Design review of the part built by this model. Coordinates are the model's own, in mm. A direction names the side the tool comes from. Coordinates: 2 decimals unless noted, no trailing zeros. Loops run counter-clockwise (first coordinate to the right, second up) from the corner with the lowest first, then second, coordinate; pieces in that order, holes last. Notation, with made-up numbers: (58.25, -18) -> (63.25, -18) arc R28 cw to (63.25, 6) -> close; hole circle Ø8 at (84, 42). An arc over 180 degrees is marked (long way). Answer in a Markdown table with one row per item.
```python
from build123d import *

# Parameters (mm, degrees)
ESQUISSE1_W             = 220
ESQUISSE1_H             = 220
ESQUISSE1_R             = 2
BOSS_EXTRU_1_DEPTH      = 4
ESQUISSE2_W             = 50
ESQUISSE2_H             = 50
ENL_V_MAT_EXTRU_1_DEPTH = 5
CONG_1_R                = 5
CHANFREIN1_SIZE         = 3
CONG_2_R                = 5


with BuildPart() as part:
    # Esquisse1 → Boss.-Extru.1 (new body)
    with BuildSketch(Plane.XY):
        with Locations((-21.875157945, -21.770833333)):
            Rectangle(ESQUISSE1_W, ESQUISSE1_H)
        with Locations((-126.875157945, 83.229166667)):
            Circle(ESQUISSE1_R, mode=Mode.SUBTRACT)
        with Locations((83.124842055, 83.229166667)):
            Circle(ESQUISSE1_R, mode=Mode.SUBTRACT)
        with Locations((-126.875157945, -126.770833333)):
            Circle(ESQUISSE1_R, mode=Mode.SUBTRACT)
        with Locations((83.124842055, -126.770833333)):
            Circle(ESQUISSE1_R, mode=Mode.SUBTRACT)
        with Locations((-113.375157945, -16.770833333)):
            Circle(ESQUISSE1_R, mode=Mode.SUBTRACT)
        with Locations((-98.375157945, -16.770833333)):
            Circle(ESQUISSE1_R, mode=Mode.SUBTRACT)
        with Locations((-113.375157945, -26.770833333)):
            Circle(ESQUISSE1_R, mode=Mode.SUBTRACT)
        with Locations((-98.375157945, -26.770833333)):
            Circle(ESQUISSE1_R, mode=Mode.SUBTRACT)
        with Locations((54.624842055, -16.770833333)):
            Circle(ESQUISSE1_R, mode=Mode.SUBTRACT)
        with Locations((69.624842055, -16.770833333)):
            Circle(ESQUISSE1_R, mode=Mode.SUBTRACT)
        with Locations((54.624842055, -26.770833333)):
            Circle(ESQUISSE1_R, mode=Mode.SUBTRACT)
        with Locations((69.624842055, -26.770833333)):
            Circle(ESQUISSE1_R, mode=Mode.SUBTRACT)
        with Locations((-21.875157945, -1.270833333)):
            Circle(ESQUISSE1_R, mode=Mode.SUBTRACT)
        with Locations((-21.875157945, -42.270833333)):
            Circle(ESQUISSE1_R, mode=Mode.SUBTRACT)
    extrude(amount=BOSS_EXTRU_1_DEPTH)

    # Esquisse2 → Enlèv. mat.-Extru.1 (cut, through all)
    with BuildSketch(Plane.XY.offset(4)):
        Polygon((-89.375157945, 53.229166667), (45.624842055, 53.229166667), (5.624842055, 13.229166667), (-49.375157945, 13.229166667), align=None)
        Polygon((-89.375157945, -96.770833333), (45.624842055, -96.770833333), (5.624842055, -56.770833333), (-49.375157945, -56.770833333), align=None)
        Polygon((88.124842055, -41.770833333), (58.124842055, -71.770833333), (58.124842055, -91.770833333), (88.124842055, -121.770833333), align=None)
        Polygon((88.124842055, 78.229166667), (88.124842055, -1.770833333), (58.124842055, 28.229166667), (58.124842055, 48.229166667), align=None)
        Polygon((-131.875157945, 78.229166667), (-131.875157945, -1.770833333), (-101.875157945, 28.229166667), (-101.875157945, 48.229166667), align=None)
        Polygon((-131.875157945, -41.770833333), (-101.875157945, -71.770833333), (-101.875157945, -91.770833333), (-131.875157945, -121.770833333), align=None)
        with Locations((18.124842055, -21.770833333)):
            Rectangle(ESQUISSE2_W, ESQUISSE2_H)
        with Locations((-61.875157945, -21.770833333)):
            Rectangle(ESQUISSE2_W, ESQUISSE2_H)
        Polygon((-121.875157945, -131.770833333), (-86.171457776, -106.770833333), (42.421141887, -106.770833333), (78.124842055, -131.770833333), align=None)
        Polygon((-121.875157945, 88.229166667), (-86.171457776, 63.229166667), (42.421141887, 63.229166667), (78.124842055, 88.229166667), align=None)
    extrude(amount=-ENL_V_MAT_EXTRU_1_DEPTH, mode=Mode.SUBTRACT)

    # Congé1
    cong_1_edges = [part.edges().sort_by_distance(p)[0] for p in [
        (-89.375157945, 53.229166667, 2),
        (45.624842055, 53.229166667, 2),
        (-89.375157945, -96.770833333, 2),
        (45.624842055, -96.770833333, 2),
    ]]
    fillet(cong_1_edges, radius=CONG_1_R)

    # Chanfrein1
    chanfrein1_edges = [part.edges().sort_by_distance(p)[0] for p in [
        (-131.875157945, 88.229166667, 2),
        (88.124842055, 88.229166667, 2),
        (88.124842055, -131.770833333, 2),
        (-131.875157945, -131.770833333, 2),
    ]]
    chamfer(chanfrein1_edges, length=CHANFREIN1_SIZE)

    # Congé2
    cong_2_edges = [part.edges().sort_by_distance(p)[0] for p in [
        (58.124842055, -91.770833333, 2),
        (58.124842055, -71.770833333, 2),
        (58.124842055, 48.229166667, 2),
        (58.124842055, 28.229166667, 2),
        (-101.875157945, 48.229166667, 2),
        (-101.875157945, 28.229166667, 2),
        (-101.875157945, -71.770833333, 2),
        (-101.875157945, -91.770833333, 2),
        (-86.875157945, -46.770833333, 2),
        (-86.875157945, 3.229166667, 2),
        (-36.875157945, 3.229166667, 2),
        (-36.875157945, -46.770833333, 2),
        (-6.875157945, -46.770833333, 2),
        (-6.875157945, 3.229166667, 2),
        (43.124842055, 3.229166667, 2),
        (43.124842055, -46.770833333, 2),
        (-86.171457776, -106.770833333, 2),
        (42.421141887, -106.770833333, 2),
        (42.421141887, 63.229166667, 2),
        (-86.171457776, 63.229166667, 2),
        (-49.375157945, 13.229166667, 2),
        (5.624842055, 13.229166667, 2),
        (-49.375157945, -56.770833333, 2),
        (5.624842055, -56.770833333, 2),
    ]]
    fillet(cong_2_edges, radius=CONG_2_R)


solid = part.part
```
(1) Tool access review of faces 5 (the flat face through (74.057, 12.297, 2.028)), 6 (the flat face through (-104.91, -119.89, 2.03)), 7 (the cylindrical face through (41.699, 1.726, 1.972)), 8 (the flat face through (-104.91, 76.35, 2.03)), 9 (the flat face through (-117.408, 63.762, 2.028)): name each direction out of +Z, -Z, +X, -X, +Y, -Y from which nothing blocks a thin tool from reaching the whole face with its end or side.
Evaluation:
| item | result |
|---|---|
| face 5 | +Z, -Z, +X |
| face 6 | +Z, -Z, -Y |
| face 7 | +Z, -Z |
| face 8 | +Z, -Z, +Y |
| face 9 | +Z, -Z, -X |
(2) Take a section at D-D on x = 15. Give the boundary of the cut face in (y, z).
Evaluation:
| item | result |
|---|---|
| outline | (-106.77, 0) -> (-96.77, 0) -> (-96.77, 4) -> (-106.77, 4) -> close; (-66.15, 0) -> (-46.77, 0) -> (-46.77, 4) -> (-66.15, 4) -> close; (3.23, 0) -> (22.6, 0) -> (22.6, 4) -> (3.23, 4) -> close; (53.23, 0) -> (63.23, 0) -> (63.23, 4) -> (53.23, 4) -> close |
(3) For pin 1 (8 mm diameter, centred on x = 42.5, y = -61, fed in from -Z); pin 2 (2.5 mm diameter, centred on x = -21.88, y = -42.27, fed in from -Z); pin 3 (2 mm diameter, centred on x = 26, z = 1.5, fed in from -Y), all flat-tipped, find the tip position at first contact; note any pin that passes through.
Evaluation:
| item | result |
|---|---|
| pin 1 | stops at z = 0 |
| pin 2 | passes through |
| pin 3 | stops at y = -106.77 |
(4) Take a section at B-B on y = -7. Give the boundary of the cut face in (x, z), and give its area (3 significant figures).
Evaluation:
| item | result |
|---|---|
| outline | (-131.88, 0) -> (-86.88, 0) -> (-86.88, 4) -> (-131.88, 4) -> close; (-36.88, 0) -> (-6.88, 0) -> (-6.88, 4) -> (-36.88, 4) -> close; (43.12, 0) -> (88.12, 0) -> (88.12, 4) -> (43.12, 4) -> close |
| area | 480 mm² |
(5) Take a section at A-A on x = -32.5. Give the boundary of the cut face in (y, z), and give its area (3 significant figures).
Evaluation:
| item | result |
|---|---|
| outline | (-106.77, 0) -> (-96.77, 0) -> (-96.77, 4) -> (-106.77, 4) -> close; (-56.77, 0) -> (13.23, 0) -> (13.23, 4) -> (-56.77, 4) -> close; (53.23, 0) -> (63.23, 0) -> (63.23, 4) -> (53.23, 4) -> close |
| area | 360 mm² |
(6) To check wall thickness, follow probe 1 along Y at (x, z) = (4, 2.1); probe 2 along Y at (x, z) = (-33.5, 0.85); probe 3 along X at (y, z) = (-33.5, 1.05). State the ranges of each line that lie inside material, in increasing order.
Evaluation:
| item | result |
|---|---|
| probe 1 | y = -106.77 to -96.77, -56.79 to -46.77, 3.23 to 13.25, 53.23 to 63.23 |
| probe 2 | y = -106.77 to -96.77, -56.77 to 13.23, 53.23 to 63.23 |
| probe 3 | x = -131.88 to -86.88, -36.88 to -6.88, 43.12 to 88.12 |
(7) Draft analysis for pull direction Y (two halves, no side actions). For faces 1 (the cylindrical face through (-85.372, 1.803, 1.972)), 2 (the flat face through (60.678, 76.013, 2.028)), 3 (the flat face through (-23, -20, 0)), 4 (the flat face through (-65.63, 29.484, 2.028)), state which applies: pulls with the +Y half, pulls with the -Y half, needs draft (parallel to the pull), parting line crosses it, or undercut.
Evaluation:
| item | result |
|---|---|
| face 1 | undercut |
| face 2 | pulls with the +Y half |
| face 3 | needs draft |
| face 4 | undercut |
(8) Take a section at C-C on y = 23. Give the boundary of the cut face in (x, z), and give its area (3 significant figures).
Evaluation:
| item | result |
|---|---|
| outline | (-107.1, 0) -> (-59.15, 0) -> (-59.15, 4) -> (-107.1, 4) -> close; (15.4, 0) -> (63.35, 0) -> (63.35, 4) -> (15.4, 4) -> close |
| area | 384 mm² |
